Check sheet for the modelled part. Datum: model origin and axes. Units: mm. Give positions to 0.01 mm unless a question says otherwise; leave off trailing zeros. Write each question's results on one line, items separated by ' | '. Start each with the question number.
1. Draft check along Y on faces 1 (the cylindrical face through (9.385, 7.514, 0.986)), 2 (the flat face through (0, 3, 0)), 3 (the cylindrical face through (-24.134, -15.934, 0.986)), 4 (the cylindrical face through (12.502, -15.127, 0.986)). Enter one of: pulls with the +Y half, pulls with the -Y half, needs draft (parallel to the pull), parting line crosses it, or undercut.
2. Go/stop test with a flat-tipped pin: pin 1 (4 mm diameter, centred on x = -15, y = -15.24, fed in from +Z). Record where the tip stops, or that it passes through.
3. Sectioned sample at A-A on x = 5.5. Give the number of separate pieces and of enclosed holes in the cut face, and give its area (3 significant figures).
4. Material ranges on line 1 along Y through (x, z) = (-8.5, 1.6); line 2 along Y through (x, z) = (13.5, 1.3); line 3 along X through (y, z) = (13.5, 1.05), recorded low to high.
```python
from build123d import *

# Parameters (mm, degrees)
F0_R     = 2.5
F1_DEPTH = 2


with BuildPart() as f1:
    # F0 (on Top) → F1 (new body)
    with BuildSketch(Plane.XY):
        with BuildLine():
            add(Edge.make_bspline(
                [(-19.704321, 21.398848), (-6.516069, 30.382996), (6.516069, 30.382996), (18.773205, 21.827396)],
                knots=[0, 0, 0, 0, 38.479913, 38.479913, 38.479913, 38.479913], degree=3))
            ThreePointArc((-19.704321, 21.398848), (-21.024547, 20.4837), (-22.054647, 19.251066))
            add(Edge.make_bspline(
                [(-22.054647, 19.251066), (-26.418865, 11.664507), (-25.900009, -6.933015), (-24.88908, -13.926778)],
                knots=[0, 0, 0, 0, 29.282142, 29.282142, 29.282142, 29.282142], degree=3))
            ThreePointArc((-24.88908, -13.926778), (-24.117585, -15.959575), (-22.556211, -17.472709))
            add(Edge.make_bspline(
                [(-10.180056, -22.870327), (-15.022858, -24.695323), (-18.484277, -19.972211), (-22.556211, -17.472709)],
                knots=[0, 0, 0, 0, 13.563984, 13.563984, 13.563984, 13.563984], degree=3))
            ThreePointArc((-10.180056, -22.870327), (0, -21.013477), (10.180056, -22.870327))
            add(Edge.make_bspline(
                [(10.180056, -22.870327), (15.022858, -24.695323), (18.484277, -19.972211), (22.556211, -17.472709)],
                knots=[0, 0, 0, 0, 13.563984, 13.563984, 13.563984, 13.563984], degree=3))
            ThreePointArc((22.556211, -17.472709), (24.117585, -15.959575), (24.88908, -13.926778))
            add(Edge.make_bspline(
                [(22.054647, 19.251066), (26.418865, 11.664507), (25.900009, -6.933015), (24.88908, -13.926778)],
                knots=[0, 0, 0, 0, 29.282142, 29.282142, 29.282142, 29.282142], degree=3))
            ThreePointArc((22.054647, 19.251066), (20.7792, 21.004476), (18.773205, 21.827396))
        make_face()
        with Locations((-15, -15.236906)):
            Circle(F0_R, mode=Mode.SUBTRACT)
        with Locations((-7, -7.236906)):
            Circle(F0_R, mode=Mode.SUBTRACT)
        with Locations((15, -15.236906)):
            Circle(F0_R, mode=Mode.SUBTRACT)
        with Locations((7, -7.236906)):
            Circle(F0_R, mode=Mode.SUBTRACT)
        with Locations((-15, 14.763094)):
            Circle(F0_R, mode=Mode.SUBTRACT)
        with Locations((-7, 6.763094)):
            Circle(F0_R, mode=Mode.SUBTRACT)
        with Locations((7, 6.763094)):
            Circle(F0_R, mode=Mode.SUBTRACT)
        with Locations((15, 14.763094)):
            Circle(F0_R, mode=Mode.SUBTRACT)
    extrude(amount=F1_DEPTH)


solid = f1.part
```
Output values:
1) face 1: undercut | face 2: needs draft | face 3: pulls with the -Y half | face 4: undercut
2) pin 1: through
3) separate pieces: 3 | enclosed holes: 0 | area: 82.4 mm2
4) line 1: -22.29 to -9.24, -5.24 to 4.76, 8.76 to 26.9 | line 2: -23.17 to -17.24, -13.24 to 12.76, 16.76 to 24.96 | line 3: -24.14 to -17.16, -12.84 to 12.84, 17.16 to 24.14
